Could you check a few things on this model? Use its own coordinates, in mm. Face numbers are marked on the shaded views. A direction names the side the tool comes from. Give positions to 0.01 mm unless a question says otherwise; leave off trailing zeros. Write each loop counter-clockwise with the first axis right and the second up, starting at its lowest first coordinate (ties: lowest second). Pieces come first, ordered by that corner, then holes. Notation, with made-up numbers: (20.5, -37.5) - (62.5, -37.5) arc R22 ccw to (62.5, -21.5) - close; hole circle Ø8 at (15, 22). An arc over 180 degrees is marked (long way). Answer in a Markdown table with one row per item.
from build123d import *

# Parameters (mm, degrees)
BOSS_EXTRUDE2_DEPTH = 3
BOSS_EXTRUDE3_DEPTH = 14
FILLET2_R           = 10
SKETCH3_R           = 1.5
BOSS_EXTRUDE4_DEPTH = 5
SKETCH2_R           = 1.5
BOSS_EXTRUDE5_DEPTH = 5


with BuildPart() as part:
    # Sketch1 → Boss-Extrude2 (new body)
    with BuildSketch(Plane(origin=(0, 0, 0), x_dir=(1, 0, 0), z_dir=(0, 1, 0))):
        with BuildLine():
            Line((-13.813102114, 29.179914519), (-13.813102114, -7.497737557))
            Line((-13.813102114, -7.497737557), (22.999876511, -7.497737557))
            ThreePointArc((22.999876511, -7.497737557), (20.393331118, -2.4896323), (15.489720926, 0.308546434))
            ThreePointArc((15.489720926, 0.308546434), (1.40152336, 8.074710364), (-6.649185051, 22.002262443))
            ThreePointArc((-6.649185051, 22.002262443), (-9.253806843, 26.566555008), (-13.813102114, 29.179914519))
        make_face()
        with BuildLine():
            Line((22.999876511, -7.497737557), (-13.813102114, -7.497737557))
            Line((-13.813102114, -7.497737557), (-13.813102114, 29.179914519))
            ThreePointArc((-13.813102114, 29.179914519), (-15.062100342, 29.421348106), (-16.331643417, 29.502262443))
            Line((-16.331643417, 29.502262443), (-16.813102114, 29.502262443))
            Line((-16.813102114, 29.502262443), (-16.813102114, -10.497737557))
            Line((-16.813102114, -10.497737557), (23.186897886, -10.497737557))
            Line((23.186897886, -10.497737557), (23.186897886, -9.422692236))
            ThreePointArc((23.186897886, -9.422692236), (23.140032725, -8.455682992), (22.999876511, -7.497737557))
        make_face()
    extrude(amount=BOSS_EXTRUDE2_DEPTH)

    # Sketch1<4> → Boss-Extrude3 (add)
    with BuildSketch(Plane(origin=(0, 0, 0), x_dir=(1, 0, 0), z_dir=(0, 1, 0))):
        with BuildLine():
            Line((22.999876511, -7.497737557), (-13.813102114, -7.497737557))
            Line((-13.813102114, -7.497737557), (-13.813102114, 29.179914519))
            ThreePointArc((-13.813102114, 29.179914519), (-15.062100342, 29.421348106), (-16.331643417, 29.502262443))
            Line((-16.331643417, 29.502262443), (-16.813102114, 29.502262443))
            Line((-16.813102114, 29.502262443), (-16.813102114, -10.497737557))
            Line((-16.813102114, -10.497737557), (23.186897886, -10.497737557))
            Line((23.186897886, -10.497737557), (23.186897886, -9.422692236))
            ThreePointArc((23.186897886, -9.422692236), (23.140032725, -8.455682992), (22.999876511, -7.497737557))
        make_face()
    extrude(amount=BOSS_EXTRUDE3_DEPTH)

    # Fillet2
    # the kernel refuses this fillet: 10 mm, written as the material it takes off along each edge
    with BuildSketch(Plane(origin=(8.668356583, 14, -29.502262443), x_dir=(0, -1, 0), z_dir=(-1, 0, 0))) as fillet2_piece_1:
        with BuildLine():
            CenterArc((FILLET2_R, FILLET2_R), FILLET2_R, 180, 90)
            Line((0, FILLET2_R), (0, 0))
            Line((0, 0), (FILLET2_R, 0))
        make_face()
    extrude(amount=50.481458697, mode=Mode.SUBTRACT)
    with BuildSketch(Plane(origin=(23.186897886, 14, 35.497737557), x_dir=(-1, 0, 0), z_dir=(0, 0, -1))) as fillet2_piece_2:
        with BuildLine():
            CenterArc((FILLET2_R, -FILLET2_R), FILLET2_R, 90, 90)
            Line((0, -FILLET2_R), (0, 0))
            Line((0, 0), (FILLET2_R, 0))
        make_face()
    extrude(amount=51.075045321, mode=Mode.SUBTRACT)

    # Sketch3 → Boss-Extrude4 (add)
    with BuildSketch(Plane.ZY.offset(16.813102114)):
        with Locations((-19.502262443, 10)):
            Circle(SKETCH3_R)
    extrude(amount=BOSS_EXTRUDE4_DEPTH)

    # Sketch4 → Revolve1 (revolve)
    with BuildSketch(Plane.ZY.offset(21.813102114)):
        with BuildLine():
            Line((-19.502262443, 12), (-19.502262443, 8))
            ThreePointArc((-19.502262443, 8), (-21.502262443, 10), (-19.502262443, 12))
        make_face()
    revolve(axis=Axis((-21.813102114, 12, -19.502262443), (0, -1, 0)))

    # Sketch2 → Boss-Extrude5 (add)
    with BuildSketch(Plane.XY.offset(10.497737557)):
        with Locations((13.186897886, 10)):
            Circle(SKETCH2_R)
    extrude(amount=BOSS_EXTRUDE5_DEPTH)

    # Sketch5 → Revolve2 (revolve)
    with BuildSketch(Plane.XY.offset(15.497737557)):
        with BuildLine():
            Line((13.186897886, 12), (13.186897886, 8))
            ThreePointArc((13.186897886, 8), (11.186897886, 10), (13.186897886, 12))
        make_face()
    revolve(axis=Axis((13.186897886, 12, 15.497737557), (0, -1, 0)))


solid = part.part
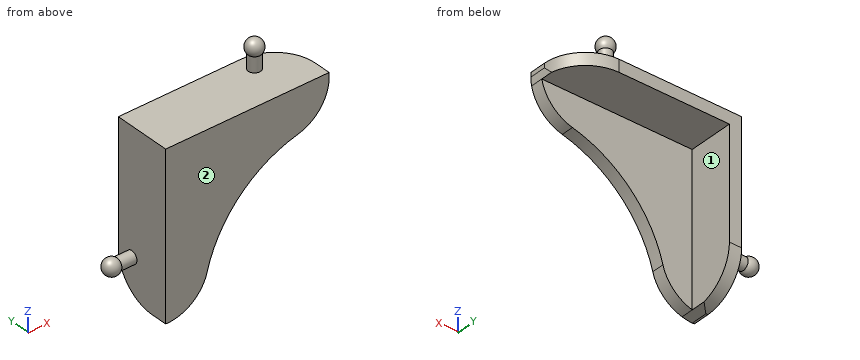
1) Will these pins go through, and if not, where does the flat tip stop? P1, Ø5.5, axis at y = 9, z = -10, coming from the +X side; P2, Ø2, axis at y = 3.5, z = 8, coming from the +X side; P3, Ø11, axis at x = 5, z = -4, coming from the +Y side.
Check values:
| item | result |
|---|---|
| P1 | stops at x = -13.81 |
| P2 | stops at x = 23.18 |
| P3 | stops at y = 3 |
2) Imagine slicing it at A-A (z = -5). List the corners of the cut face in (x, y) for me.
Check values:
| item | result |
|---|---|
| outline | (-16.81, 0) - (5.09, 0) - (5.09, 3) - (-13.81, 3) - (-13.81, 14) - (-16.81, 14) - close |
3) Imagine slicing it at C-C (y = 10). List the corners of the cut face in (x, z) for me, then the cut area to 3 significant figures.
Check values:
| item | result |
|---|---|
| outline | (-20.49, -21) - (-16.81, -21) - (-16.81, -27.5) - (-13.81, -27.5) - (-13.81, 7.5) - (21.19, 7.5) - (21.19, 10.5) - (14.69, 10.5) - (14.69, 14.17) arc R2 ccw (long way) to (11.69, 14.17) - (11.69, 10.5) - (-16.81, 10.5) - (-16.81, -18) - (-20.49, -18) arc R2 ccw (long way) to start |
| area | 263 mm2 |
4) Imagine slicing it at B-B (x = -9). List the corners of the cut face in (y, z) for me, then the cut area to 3 significant figures.
Check values:
| item | result |
|---|---|
| outline | (0, -26.3) - (3, -26.3) - (3, 7.5) - (14, 7.5) - (14, 10.5) - (0, 10.5) - close |
| area | 143 mm2 |
5) If I drill on line 1 (X direction, y = 11, z = -7); line 2 (Y direction, x = -13.5, z = 0.5); line 3 (Z direction, x = 9, y = 5.25), over which ranges is the centre line in solid material (lowest first)?
Check values:
| item | result |
|---|---|
| line 1 | x = -16.81 to -13.81 |
| line 2 | y = 0 to 3 |
| line 3 | z = 7.5 to 10.5 |
6) On a 3-axis mill with a long thin cutter (end or side, diameter ignored), from which of +Z, -Z, +X, -X, +Y, -Y can I reach the whole of each face in a straight line? I mean the marked faces 1 and 2. Say none if no direction works.
Check values:
| item | result |
|---|---|
| face 1 | -Z, +X, +Y |
| face 2 | +Z, -Z, +X, -X, -Y |
